Source: CAD feature listing. Evaluate the final solid. Frame: model axes, mm. A direction names the side the tool comes from. Round coordinates to 2 decimals unless told otherwise and drop trailing zeros. Loops run counter-clockwise (first coordinate to the right, second up) from the corner with the lowest first, then second, coordinate; pieces in that order, holes last. Notation, with made-up numbers: M -19,29.5 L 9,29.5 A37 cw 9,66.5 Z; hole C 43.5,86.5 d8. An arc over 180 degrees is marked long. Write each question's results on one line, items separated by ' | '. Start each with the question number.
1. Ray query, line 1 (X direction, y = 21.5, z = 26); line 2 (Y direction, x = -24, z = 51); line 3 (Y direction, x = -22.5, z = 45). Return the intervals inside material, ascending.
2. Section A-A on x = -21.25. Output: boundary loops of the cut face in (y, z), and give its area (3 significant figures).
3. Set-up query: faces 1 (the flat face through (-18.57, 23.1, 34.51)), 2 (the flat face through (-22, 27.328, 35)), 3 (the flat face through (-21, 23.328, 35)). Return all of +Z, -Z, +X, -X, +Y, -Y with unobstructed straight access to the full face (end or side cutting, diameter ignored); none if empty.
4. Contact query for flat-ended pins moving along their axis: pin 1 Ø1 at (x, y) = (-19, 28) entering from -Z; pin 2 Ø1.9 at (x, z) = (-22, 41.5) entering from -Y; pin 3 Ø1.2 at (y, z) = (25, 26) entering from +X; pin 4 Ø1.2 at (x, z) = (-21, 44.5) entering from +Y. Output: stop coordinate, or through.
5. Section B-B on y = 25. Output: boundary loops of the cut face in (x, z), and give its area (3 significant figures).
6. Draft query along X for faces 4 (the flat face through (-21, 25, 70)), 5 (the flat face through (-23.74, 22.39, 34.51)), 6 (the flat face through (-19.508, 25, 35)). Return one class per face: released by +X, released by -X, zero draft, split by the parting line, or undercut.
from build123d import *

# Parameters (mm, degrees)
BOSS_EXTRUDE1_DEPTH = 70


with BuildPart() as part:
    # Sketch1 → Boss-Extrude1 (new body)
    with BuildSketch(Plane.XY):
        with BuildLine():
            Line((-26.434620061, 28.496491655), (-25.979594809, 28.951516907))
            ThreePointArc((-25.979594809, 28.951516907), (-25.906371503, 29.128293603), (-25.979594808, 29.305070299))
            Line((-25.979594808, 29.305070299), (-26.43462006, 29.760095551))
            ThreePointArc((-26.43462006, 29.760095551), (-26.488813248, 29.841201388), (-26.507843365, 29.936872247))
            Line((-26.507843365, 29.936872247), (-26.507843365, 30.078293605))
            ThreePointArc((-26.507843365, 30.078293605), (-26.43462006, 30.255070299), (-26.257843366, 30.328293604))
            Line((-26.257843366, 30.328293604), (-26.11642201, 30.328293604))
            ThreePointArc((-26.11642201, 30.328293604), (-26.020751153, 30.309263487), (-25.939645316, 30.255070299))
            Line((-25.939645316, 30.255070299), (-25.484620061, 29.800045045))
            ThreePointArc((-25.484620061, 29.800045045), (-25.307843366, 29.72682174), (-25.131066671, 29.800045045))
            Line((-25.131066671, 29.800045045), (-24.676041418, 30.255070298))
            ThreePointArc((-24.676041418, 30.255070298), (-24.594935581, 30.309263487), (-24.499264722, 30.328293604))
            Line((-24.499264722, 30.328293604), (-24.042157942, 30.328293604))
            ThreePointArc((-24.042157942, 30.328293604), (-23.949769989, 30.266561947), (-23.971447265, 30.157582926))
            Line((-23.971447265, 30.157582926), (-24.623959891, 29.505070299))
            ThreePointArc((-24.623959891, 29.505070299), (-24.697183196, 29.328293604), (-24.623959891, 29.15151691))
            Line((-24.623959891, 29.15151691), (-22.873959891, 27.401516909))
            ThreePointArc((-22.873959891, 27.401516909), (-22.792854054, 27.347323722), (-22.697183196, 27.328293605))
            Line((-22.697183196, 27.328293605), (-20.318503539, 27.328293605))
            ThreePointArc((-20.318503539, 27.328293605), (-20.222832681, 27.347323722), (-20.141726844, 27.401516909))
            Line((-20.141726844, 27.401516909), (-18.391726844, 29.15151691))
            ThreePointArc((-18.391726844, 29.15151691), (-18.318503539, 29.328293604), (-18.391726844, 29.505070299))
            Line((-18.391726844, 29.505070299), (-19.04423947, 30.157582926))
            ThreePointArc((-19.04423947, 30.157582926), (-19.065916745, 30.266561947), (-18.973528793, 30.328293604))
            Line((-18.973528793, 30.328293604), (-18.516422013, 30.328293604))
            ThreePointArc((-18.516422013, 30.328293604), (-18.420751155, 30.309263487), (-18.339645319, 30.2550703))
            Line((-18.339645319, 30.2550703), (-17.884620064, 29.800045045))
            ThreePointArc((-17.884620064, 29.800045045), (-17.707843369, 29.72682174), (-17.531066674, 29.800045045))
            Line((-17.531066674, 29.800045045), (-17.07604142, 30.2550703))
            ThreePointArc((-17.07604142, 30.2550703), (-16.994935583, 30.309263487), (-16.899264725, 30.328293604))
            Line((-16.899264725, 30.328293604), (-16.75784337, 30.328293604))
            ThreePointArc((-16.75784337, 30.328293604), (-16.581066675, 30.255070299), (-16.507843371, 30.078293605))
            Line((-16.507843371, 30.078293605), (-16.507843371, 29.936872247))
            ThreePointArc((-16.507843371, 29.936872247), (-16.526873488, 29.841201389), (-16.581066675, 29.760095552))
            Line((-16.581066675, 29.760095552), (-17.036091927, 29.3050703))
            ThreePointArc((-17.036091927, 29.3050703), (-17.109315232, 29.128293603), (-17.036091926, 28.951516907))
            Line((-17.036091926, 28.951516907), (-16.581066674, 28.496491655))
            ThreePointArc((-16.581066674, 28.496491655), (-16.526873486, 28.415385818), (-16.507843369, 28.31971496))
            Line((-16.507843369, 28.31971496), (-16.507843369, 27.862608178))
            ThreePointArc((-16.507843369, 27.862608178), (-16.569575025, 27.770220231), (-16.678554041, 27.791897499))
            Line((-16.678554041, 27.791897499), (-17.331066668, 28.444410126))
            ThreePointArc((-17.331066668, 28.444410126), (-17.507843364, 28.517633431), (-17.68462006, 28.444410125))
            Line((-17.68462006, 28.444410125), (-19.434620061, 26.694410125))
            ThreePointArc((-19.434620061, 26.694410125), (-19.488813248, 26.613304288), (-19.507843364, 26.51763343))
            Line((-19.507843364, 26.51763343), (-19.507843364, 24.138953775))
            ThreePointArc((-19.507843364, 24.138953775), (-19.488813247, 24.043282917), (-19.434620059, 23.962177079))
            Line((-19.434620059, 23.962177079), (-17.684620059, 22.212177079))
            ThreePointArc((-17.684620059, 22.212177079), (-17.507843363, 22.138953773), (-17.331066666, 22.212177077))
            Line((-17.331066666, 22.212177077), (-16.67855404, 22.864689704))
            ThreePointArc((-16.67855404, 22.864689704), (-16.569575019, 22.886366979), (-16.507843363, 22.793979027))
            Line((-16.507843363, 22.793979027), (-16.507843363, 22.336872245))
            ThreePointArc((-16.507843363, 22.336872245), (-16.52687348, 22.241201387), (-16.581066668, 22.16009555))
            Line((-16.581066668, 22.16009555), (-17.036091921, 21.705070296))
            ThreePointArc((-17.036091921, 21.705070296), (-17.109315225, 21.528293601), (-17.036091921, 21.351516906))
            Line((-17.036091921, 21.351516906), (-16.581066669, 20.896491654))
            ThreePointArc((-16.581066669, 20.896491654), (-16.526873481, 20.815385817), (-16.507843364, 20.719714959))
            Line((-16.507843364, 20.719714959), (-16.507843364, 20.578293601))
            ThreePointArc((-16.507843364, 20.578293601), (-16.581066669, 20.401516906), (-16.757843364, 20.328293601))
            Line((-16.757843364, 20.328293601), (-16.89926472, 20.328293601))
            ThreePointArc((-16.89926472, 20.328293601), (-16.994935578, 20.347323718), (-17.076041415, 20.401516905))
            Line((-17.076041415, 20.401516905), (-17.53106667, 20.85654216))
            ThreePointArc((-17.53106667, 20.85654216), (-17.707843365, 20.929765464), (-17.88462006, 20.85654216))
            Line((-17.88462006, 20.85654216), (-18.339645314, 20.401516905))
            ThreePointArc((-18.339645314, 20.401516905), (-18.420751151, 20.347323718), (-18.516422009, 20.328293601))
            Line((-18.516422009, 20.328293601), (-18.973528789, 20.328293601))
            ThreePointArc((-18.973528789, 20.328293601), (-19.065916743, 20.390025258), (-19.044239468, 20.499004281))
            Line((-19.044239468, 20.499004281), (-18.391726841, 21.151516907))
            ThreePointArc((-18.391726841, 21.151516907), (-18.318503536, 21.328293602), (-18.391726841, 21.505070297))
            Line((-18.391726841, 21.505070297), (-20.141726841, 23.255070297))
            ThreePointArc((-20.141726841, 23.255070297), (-20.222832678, 23.309263485), (-20.318503536, 23.328293602))
            Line((-20.318503536, 23.328293602), (-22.697183193, 23.328293602))
            ThreePointArc((-22.697183193, 23.328293602), (-22.792854051, 23.309263485), (-22.873959889, 23.255070297))
            Line((-22.873959889, 23.255070297), (-24.623959889, 21.505070297))
            ThreePointArc((-24.623959889, 21.505070297), (-24.697183193, 21.328293602), (-24.623959889, 21.151516907))
            Line((-24.623959889, 21.151516907), (-23.971447262, 20.499004281))
            ThreePointArc((-23.971447262, 20.499004281), (-23.949769986, 20.390025258), (-24.042157941, 20.328293601))
            Line((-24.042157941, 20.328293601), (-24.49926472, 20.328293601))
            ThreePointArc((-24.49926472, 20.328293601), (-24.594935579, 20.347323718), (-24.676041417, 20.401516907))
            Line((-24.676041417, 20.401516907), (-25.131066671, 20.85654216))
            ThreePointArc((-25.131066671, 20.85654216), (-25.307843365, 20.929765464), (-25.48462006, 20.85654216))
            Line((-25.48462006, 20.85654216), (-25.939645315, 20.401516906))
            ThreePointArc((-25.939645315, 20.401516906), (-26.020751152, 20.347323718), (-26.11642201, 20.328293601))
            Line((-26.11642201, 20.328293601), (-26.257843366, 20.328293601))
            ThreePointArc((-26.257843366, 20.328293601), (-26.434620061, 20.401516906), (-26.507843366, 20.578293601))
            Line((-26.507843366, 20.578293601), (-26.507843366, 20.719714959))
            ThreePointArc((-26.507843366, 20.719714959), (-26.488813249, 20.815385817), (-26.434620061, 20.896491655))
            Line((-26.434620061, 20.896491655), (-25.979594809, 21.351516907))
            ThreePointArc((-25.979594809, 21.351516907), (-25.906371505, 21.528293602), (-25.979594809, 21.705070297))
            Line((-25.979594809, 21.705070297), (-26.434620063, 22.16009555))
            ThreePointArc((-26.434620063, 22.16009555), (-26.48881325, 22.241201387), (-26.507843367, 22.336872245))
            Line((-26.507843367, 22.336872245), (-26.507843367, 22.793979027))
            ThreePointArc((-26.507843367, 22.793979027), (-26.446111711, 22.88636698), (-26.337132691, 22.864689705))
            Line((-26.337132691, 22.864689705), (-25.684620064, 22.212177078))
            ThreePointArc((-25.684620064, 22.212177078), (-25.507843369, 22.138953774), (-25.331066674, 22.212177078))
            Line((-25.331066674, 22.212177078), (-23.581066674, 23.962177078))
            ThreePointArc((-23.581066674, 23.962177078), (-23.526873485, 24.043282916), (-23.507843368, 24.138953775))
            Line((-23.507843368, 24.138953775), (-23.507843368, 26.51763343))
            ThreePointArc((-23.507843368, 26.51763343), (-23.526873484, 26.613304288), (-23.581066672, 26.694410125))
            Line((-23.581066672, 26.694410125), (-25.331066672, 28.444410125))
            ThreePointArc((-25.331066672, 28.444410125), (-25.507843367, 28.51763343), (-25.684620062, 28.444410125))
            Line((-25.684620062, 28.444410125), (-26.337132689, 27.791897498))
            ThreePointArc((-26.337132689, 27.791897498), (-26.44611171, 27.770220225), (-26.507843366, 27.862608178))
            Line((-26.507843366, 27.862608178), (-26.507843366, 28.31971496))
            ThreePointArc((-26.507843366, 28.31971496), (-26.488813249, 28.415385818), (-26.434620061, 28.496491655))
        make_face()
    extrude(amount=BOSS_EXTRUDE1_DEPTH)


solid = part.part
Taken from the geometry:
1) line 1: -25.91 to -24.63, -18.39 to -17.11 | line 2: 20.34 to 20.53, 22.13 to 23.54, 27.11 to 28.53, 30.13 to 30.32 | line 3: 23.33 to 27.33
2) outline: M 23.33,0 L 27.33,0 L 27.33,70 L 23.33,70 Z | area: 280 mm^2
3) face 1: +Z, -Z | face 2: +Z, -Z, +Y | face 3: +Z, -Z, -Y
4) pin 1: z = 0 | pin 2: y = 23.18 | pin 3: x = -19.51 | pin 4: y = 27.33
5) outline: M -23.51,0 L -19.51,0 L -19.51,70 L -23.51,70 Z | area: 280 mm^2
6) face 4: zero draft | face 5: undercut | face 6: released by +X
